```python
from build123d import *

# Parameters (mm, degrees)
BOSS_EXTRUDE1_DEPTH     = 381
CUT_EXTRUDE3_DEPTH      = 383.403015687
CUT_EXTRUDE3_DEPTH_BACK = 383.403015687
CUT_EXTRUDE4_REACH      = 384.403
SKETCH6_R               = 3.175
CUT_EXTRUDE5_REACH      = 384.69
SKETCH7_R               = 3.175
CUT_EXTRUDE6_REACH      = 384.403
SKETCH8_R               = 3.175


with BuildPart() as part:
    # Sketch1 → Boss-Extrude1 (new body)
    with BuildSketch(Plane.XY):
        Polygon((0, 0), (0, -25.4), (-25.4, -25.4), (-25.4, -20.6375), (-4.7625, -20.6375), (-4.7625, 0), align=None)
    extrude(amount=BOSS_EXTRUDE1_DEPTH)

    # Sketch4 → Cut-Extrude3 (cut, two sides: drawn at the far end of the back side and taken through both)
    with BuildSketch(Plane.ZY.offset(4.7625).offset(-CUT_EXTRUDE3_DEPTH_BACK)):
        Polygon((1030.877066877, -439.409233154), (381, -20.6375), (348.97339241, 0), (-300.903674467, 418.771733154), (536.63979184, 1718.525866908), (1868.420533185, 860.3449006), align=None)
    extrude(amount=CUT_EXTRUDE3_DEPTH + CUT_EXTRUDE3_DEPTH_BACK, mode=Mode.SUBTRACT)

    # Sketch6 → Cut-Extrude4 (cut, up to next)
    with BuildSketch(Plane.ZY.offset(4.7625), mode=Mode.PRIVATE) as cut_extrude4_sk1:
        with Locations((6.35, -15.875)):
            Circle(SKETCH6_R)
    cut_extrude4_tool1 = extrude(cut_extrude4_sk1.sketch, amount=-CUT_EXTRUDE4_REACH, mode=Mode.PRIVATE) & part.part
    # Sketch6 → Cut-Extrude4 (cut, up to next)
    with BuildSketch(Plane.ZY.offset(4.7625), mode=Mode.PRIVATE) as cut_extrude4_sk2:
        with Locations((12.7, -6.35)):
            Circle(SKETCH6_R)
    cut_extrude4_tool2 = extrude(cut_extrude4_sk2.sketch, amount=-CUT_EXTRUDE4_REACH, mode=Mode.PRIVATE) & part.part
    add(cut_extrude4_tool1.solids().sort_by_distance((-4.7625, -15.875, 6.35))[0], mode=Mode.SUBTRACT)
    add(cut_extrude4_tool2.solids().sort_by_distance((-4.7625, -6.35, 12.7))[0], mode=Mode.SUBTRACT)

    # Sketch7 → Cut-Extrude5 (cut, up to next)
    with BuildSketch(Plane(origin=(0, 0, 0), x_dir=(0, 0, -1), z_dir=(1, 0, 0)), mode=Mode.PRIVATE) as cut_extrude5_sk1:
        with Locations(Location((-107.490701513, -11.929615818, 0), (0, 0, 90))):
            Circle(SKETCH7_R)
    cut_extrude5_tool1 = extrude(cut_extrude5_sk1.sketch, amount=-CUT_EXTRUDE5_REACH, mode=Mode.PRIVATE) & part.part
    add(cut_extrude5_tool1.solids().sort_by_distance((0, -11.929616, 107.490702))[0], mode=Mode.SUBTRACT)

    # Sketch8 → Cut-Extrude6 (cut, up to next)
    with BuildSketch(Plane(origin=(0, -20.6375, 0), x_dir=(1, 0, 0), z_dir=(0, 1, 0)), mode=Mode.PRIVATE) as cut_extrude6_sk1:
        with Locations(Location((-15.08125, -12.7, 0), (0, 0, 180))):
            Circle(SKETCH8_R)
    cut_extrude6_tool1 = extrude(cut_extrude6_sk1.sketch, amount=-CUT_EXTRUDE6_REACH, mode=Mode.PRIVATE) & part.part
    add(cut_extrude6_tool1.solids().sort_by_distance((-15.08125, -20.6375, 12.7))[0], mode=Mode.SUBTRACT)


solid = part.part
```
The model under review builds one solid part; all positions refer to its coordinate system, in mm. Coordinates: 2 decimals unless noted, no trailing zeros. Write each loop counter-clockwise with the first axis right and the second up, starting at its lowest first coordinate (ties: lowest second). Pieces come first, ordered by that corner, then holes. Notation, with made-up numbers: (1.5, -26.5) - (35.5, -26.5) arc R6 cw to (35.5, -22.5) - close; hole circle Ø11 at (60.25, 27.25). An arc over 180 degrees is marked (long way). Answer in a Markdown table with one row per item. Add a question column.
Q1. To check wall thickness, follow line 1 along Y through (x, z) = (-1.85, 6.35); line 2 along X through (y, z) = (-6.5, 104.5); line 3 along Y through (x, z) = (-12, 32). State the ranges of each line that lie inside material, in increasing order. Write a range as from..to.
Q2. Consider section B-B on z = 287.5. Give the boundary of the cut face in (x, y).
Q3. Consider section A-A on z = 12.7. Give the boundary of the cut face in (x, y) (1 decimal), then the cut area to 3 significant figures.
Q4. Consider section C-C on x = -21.5. Give the boundary of the cut face in (y, z), then the cut area to 3 significant figures.
Q5. Clearance check with flat-ended pins moving along their axes: pin 1 (6 mm diameter, centred on x = -18, z = 229.5, fed in from +Y); pin 2 (7.5 mm diameter, centred on y = -15.875, z = 6.35, fed in from -X). State where each tip first meets the part, or that it passes through.
Q6. Draft analysis for pull direction Y (two halves, no side actions). For faces 1 (the face through (-4.762, -10, 188)), 2 (the face through (-2.41, -8.28, 10.18)), 3 (the face through (-2.35, -12.62, 104.39)), 4 (the face through (-15, -20.638, 188)), state which applies: +Y half, -Y half, draft (parallel to the pull), parting line (faces both ways), or undercut.
Answers below:
| question | item | result |
|---|---|---|
| 1 | line 1 | -25.4..-19.05, -12.7..0 |
| 1 | line 2 | -4.76..0 |
| 1 | line 3 | -25.4..-20.64 |
| 2 | outline | (-25.4, -25.4) - (0, -25.4) - (0, 0) - (-4.76, 0) - (-4.76, -20.64) - (-25.4, -20.64) - close |
| 3 | outline | (-25.4, -25.4) - (-18.3, -25.4) - (-18.3, -20.6) - (-25.4, -20.6) - close; (-11.9, -25.4) - (0, -25.4) - (0, -9.5) - (-4.8, -9.5) - (-4.8, -20.6) - (-11.9, -20.6) - close; (-4.8, -3.2) - (0, -3.2) - (0, 0) - (-4.8, 0) - close |
| 3 | area | 159 mm² |
| 4 | outline | (-25.4, 0) - (-20.64, 0) - (-20.64, 381) - (-25.4, 381) - close |
| 4 | area | 1,810 mm² |
| 5 | pin 1 | y = -20.64 |
| 5 | pin 2 | x = -4.76 |
| 6 | face 1 | draft |
| 6 | face 2 | undercut |
| 6 | face 3 | undercut |
| 6 | face 4 | +Y half |
